Autodesk Inventor part; units mm, degrees
ref_plane "YZ Plane" through (0, 0, 0) normal (1, 0, 0) x (0, 1, 0)
ref_plane "XZ Plane" through (0, 0, 0) normal (0, 1, 0) x (-1, 0, 0)
ref_plane "XY Plane" through (0, 0, 0) normal (0, 0, 1) x (1, 0, 0)
sketch "Sketch1" plane through (0, 0, 0) normal (0, 0, 1) x (1, 0, 0)
  line L0 (-7.0069, 50.8) -> (7.0069, 50.8)
  line L1 (7.0069, 50.8) -> (7.0069, 0)
  line L2 (7.0069, 0) -> (-7.0069, 0)
  line L3 (-7.0069, 0) -> (-7.0069, 50.8)
  line L4 (7.0069, 34.925) -> (32.4069, 34.925)
  line L5 (7.0069, 19.05) -> (32.4069, 19.05)
  arc A0 (32.4069, 19.05) -> (32.4069, 34.925) centre (32.4069, 26.9875) ccw
  line L6 (7.0069, 38.1) -> (32.4069, 38.1)
  line L7 (7.9386, 15.8944) -> (31.7511, 15.8944)
  arc A1 (31.7511, 15.8944) -> (32.4069, 38.1) centre (32.4069, 26.9875) ccw
  line L8 (7.9386, 15.8944) -> (7.0069, 15.8944)
  point P0 (0, 0)
  dimension "d0" = 50.8
  dimension "d1" = 25.4
extrude "Extrusion1" add sketch "Sketch1" along normal blind 76.2 contours L0 L1 L2 L3 | L6 A1 L7 L8 L1 L5 A0 L4
properties part number "WireHolder"
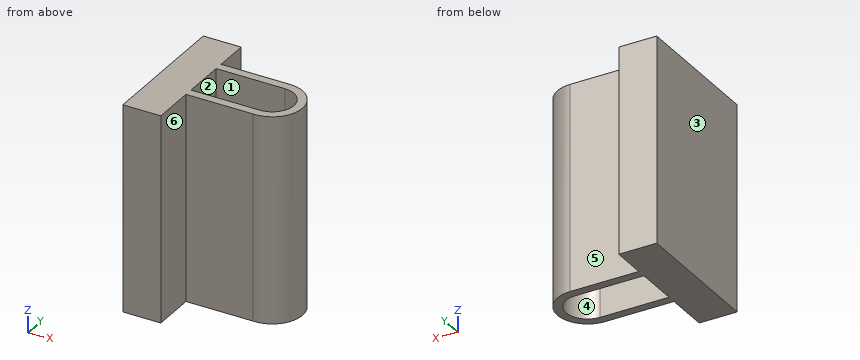
Geometry check sheet. Reference: the model listing, model coordinates, mm. Face numbers are marked on the shaded views. A direction names the side the tool comes from. Round coordinates to 2 decimals unless told otherwise and drop trailing zeros. Write each loop counter-clockwise with the first axis right and the second up, starting at its lowest first coordinate (ties: lowest second). Pieces come first, ordered by that corner, then holes.
Item 1: Material ranges on line 1 along Y through (x, z) = (20.5, 60) (3 decimals); line 2 along X through (y, z) = (43.5, 59.5); line 3 along Y through (x, z) = (33.5, 29.5), recorded low to high.
Determined:
line 1: y = 15.894 to 19.05, 34.925 to 38.1
line 2: x = -7.01 to 7.01
line 3: y = 15.93 to 19.13, 34.85 to 38.05
Item 2: Section check D-D (y = 3.5). Record the boundary of the cut face in (x, z), plus the area to 3 significant figures.
Determined:
outline: (-7.01, 0) - (7.01, 0) - (7.01, 76.2) - (-7.01, 76.2) - close
area: 1,070 mm2
Item 3: Go/stop test with flat-tipped pins: pin 1 Ø5 at (y, z) = (9.5, 25.5) entering from +X; pin 2 Ø20 at (x, z) = (16.5, 27) entering from -Y; pin 3 Ø1 at (x, z) = (19, 46.5) entering from +Y; pin 4 Ø1.5 at (x, z) = (21.5, 20) entering from -Y. Record where each tip stops, or that it passes through.
Determined:
pin 1: stops at x = 7.01
pin 2: stops at y = 0
pin 3: stops at y = 38.1
pin 4: stops at y = 15.89
Item 4: Section check A-A (x = 18.5). Record the boundary of the cut face in (y, z) (3 decimals).
Determined:
outline: (15.894, 0) - (19.05, 0) - (19.05, 76.2) - (15.894, 76.2) - close; (34.925, 0) - (38.1, 0) - (38.1, 76.2) - (34.925, 76.2) - close
Item 5: Section check B-B (y = 24). Record the boundary of the cut face in (x, z), plus the area to 3 significant figures.
Determined:
outline: (-7.01, 0) - (7.01, 0) - (7.01, 76.2) - (-7.01, 76.2) - close; (39.76, 0) - (43.11, 0) - (43.11, 76.2) - (39.76, 76.2) - close
area: 1,320 mm2
Item 6: Mould release check, pull along X, two halves, no side actions. Record for the marked faces 1, 2 and 3: +X half, -X half, draft (parallel to the pull), parting line (faces both ways), or undercut.
Determined:
face 1: undercut
face 2: undercut
face 3: -X half
Item 7: Access from +Z, -Z, +X, -X, +Y, -Y to the whole of each face (thin tool, end or side, straight path). Record for the marked faces 4, 5 and 6.
Determined:
face 4: +Z, -Z
face 5: +Z, -Z, +X, +Y
face 6: +Z, -Z, +X, -Y
